Geometry check sheet. Reference: drawing and pictorial views, mm from the part's lowest x, y, z. A direction names the side the tool comes from. Coordinates: 2 decimals unless noted, no trailing zeros. Loops run counter-clockwise (first coordinate to the right, second up) from the corner with the lowest first, then second, coordinate; pieces in that order, holes last. Notation, with made-up numbers: (64.25, 17) - (70.25, 17) arc R10 cw to (70.25, 34) - close; hole circle Ø2 at (28, 38). An arc over 180 degrees is marked (long way). Write each question's results on one line, items separated by ' | '. Start each with the question number.
1. Tool access check on the marked faces 1, 2 and 3. Record the directions out of +Z, -Z, +X, -X, +Y, -Y that give a thin tool (end or side, any length) a straight path to the whole face; none if there is none.
2. Cross-section at A-A (y = 18). Record the cut outline in (x, z), and give its area (3 significant figures).
3. Draft check along Y on the marked faces 4, 5, 6 and 7. Enter one of: released by +Y, released by -Y, zero draft, split by the parting line, or undercut.
4. Cross-section at B-B (z = 2.25). Record the cut outline in (x, y), and give its area (3 significant figures).
5. Cross-section at D-D (x = 78.5). Record the cut outline in (y, z).
6. Cross-section at C-C (x = 42). Record the cut outline in (y, z).
7. Thickness scan on line 1 (X direction, y = 15, z = 4); line 2 (X direction, y = 24.5, z = 2.25); line 3 (Y direction, x = 81.5, z = 7). Record the ranges inside material, lowest first. Write a range as [from, to].
8. Gauge pin test, flat ends, axial feed: P1, Ø5, axis at x = 17.5, z = 6, coming from the -Y side; P2, Ø2, axis at y = 26.5, z = 4, coming from the -X side; P3, Ø3, axis at x = 23, z = 4, coming from the +Y side. Record the tip position at first contact, or that the pin passes through.
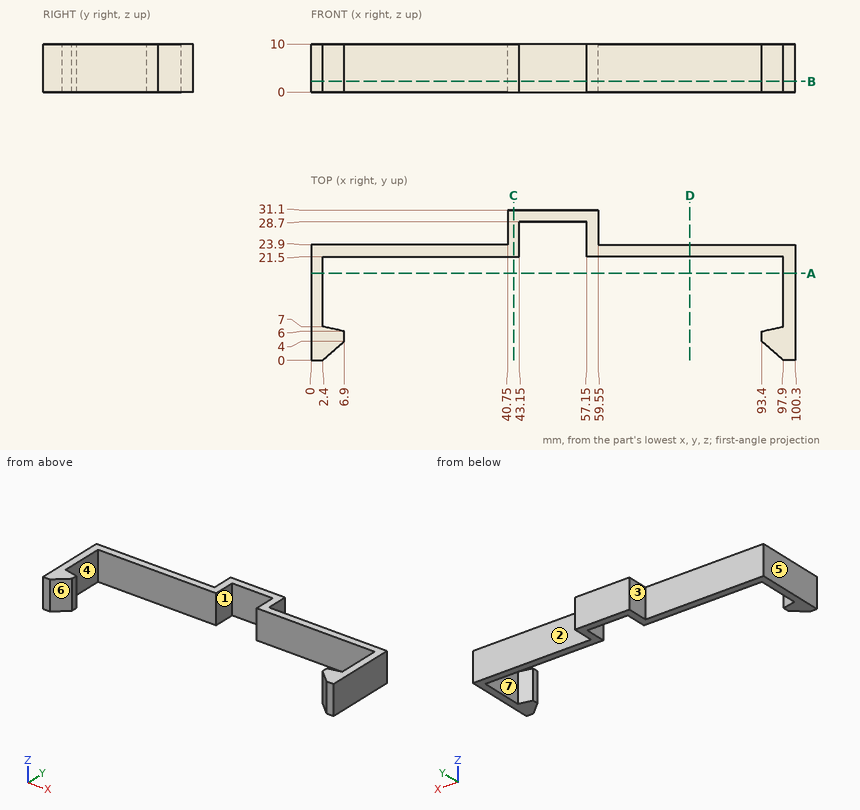
Established:
1) face 1: +Z, -Z, -Y | face 2: +Z, -Z, +X, +Y | face 3: +Z, -Z, -X, +Y
2) outline: (0, 0) - (2.4, 0) - (2.4, 10) - (0, 10) - close; (97.9, 0) - (100.3, 0) - (100.3, 10) - (97.9, 10) - close | area: 48.0 mm^2
3) face 4: undercut | face 5: zero draft | face 6: released by -Y | face 7: undercut
4) outline: (0, 0) - (2.4, 0) - (6.9, 4) - (6.9, 6) - (2.4, 7) - (2.4, 21.5) - (43.15, 21.5) - (43.15, 28.7) - (57.15, 28.7) - (57.15, 21.5) - (97.9, 21.5) - (97.9, 7) - (93.4, 6) - (93.4, 4) - (97.9, 0) - (100.3, 0) - (100.3, 23.9) - (59.55, 23.9) - (59.55, 31.1) - (40.75, 31.1) - (40.75, 23.9) - (0, 23.9) - close | area: 419 mm^2
5) outline: (21.5, 0) - (23.9, 0) - (23.9, 10) - (21.5, 10) - close
6) outline: (21.5, 0) - (31.1, 0) - (31.1, 10) - (21.5, 10) - close
7) line 1: [0, 2.4], [97.9, 100.3] | line 2: [40.75, 43.15], [57.15, 59.55] | line 3: [21.5, 23.9]
8) P1: y = 21.5 | P2: x = 40.75 | P3: y = 23.9
